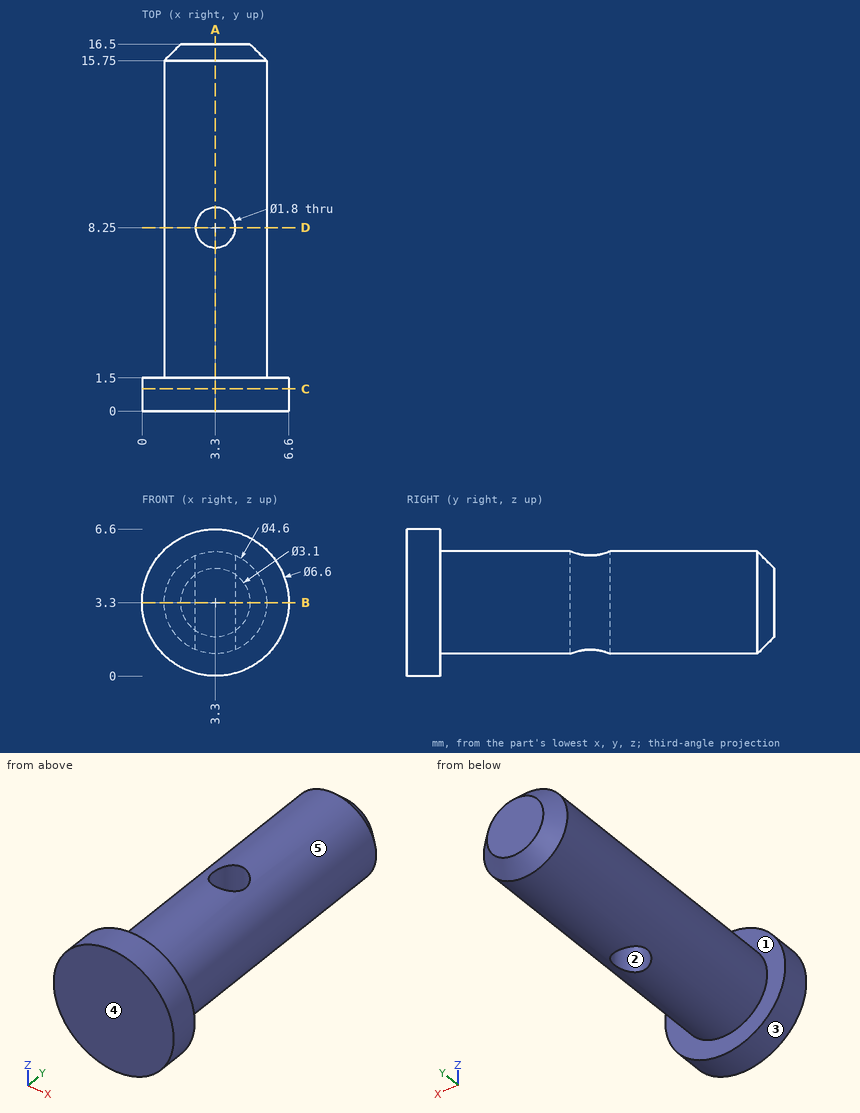
Study the drawing (mm; zero at the part's minimum x, y, z) and answer. A direction names the side the tool comes from. Coordinates: 2 decimals unless noted, no trailing zeros. Loops run counter-clockwise (first coordinate to the right, second up) from the corner with the lowest first, then second, coordinate; pieces in that order, holes last. Notation, with made-up numbers: M -11,-27 L 27,-27 A22 cw 27,-16 Z; hole C -15.5,12 d2. An arc over 180 degrees is marked long. Answer in a Markdown table with one row per item. Add a question column.
1. Find section B-B, the plane z = 3.3. Write down the section's boundary in (x, y).
2. Find section C-C, the plane y = 1. Write down the section's boundary in (x, z).
3. The mould has two halves that part along X. Classify the marked faces 1, 2 and 3: pulls with the +X half, pulls with the -X half, needs draft (parallel to the pull), parting line crosses it, or undercut.
4. Flat-ended cylindrical pins translate along their axes: P1, Ø1.5, axis at y = 14.5, z = 2.5, coming from the -X side; P2, Ø1.5, axis at x = 5, z = 3.5, coming from the +Y side; P3, Ø1.5, axis at y = 5.5, z = 0.5, coming from the -X side; P4, Ø2, axis at x = 4, y = 12, coming from the +Z side. Find the tip coordinate at first contact, or state that the pin passes through.
5. Find section A-A, the plane x = 3.3. Write down the section's boundary in (y, z).
6. Find section D-D, the plane y = 8.25. Write down the section's boundary in (x, z), then the cut area to 3 significant figures.
7. A tool of negligible diameter and unlimited length cuts with its end or side. For the marked faces 4 and 5, from which of +Z, -Z, +X, -X, +Y, -Y can it reach the whole face along a straight path? Write none if from no direction.
8. Consider L1, parallel to Y at x = 3.3, z = 4.3; L2, parallel to Y at x = 1, z = 2; L3, parallel to X at y = 7.75, z = 3. Determine where each line is inside the solid, lowest interval first.
Reported:
| question | item | result |
|---|---|---|
| 1 | outline | M 0,0 L 6.6,0 L 6.6,1.5 L 5.6,1.5 L 5.6,15.75 L 4.85,16.5 L 1.75,16.5 L 1,15.75 L 1,1.5 L 0,1.5 Z; hole C 3.3,8.25 d1.8 |
| 2 | outline | C 3.3,3.3 d6.6 |
| 3 | face 1 | needs draft |
| 3 | face 2 | undercut |
| 3 | face 3 | parting line crosses it |
| 4 | P1 | stops at x = 1 |
| 4 | P2 | stops at y = 16.5 |
| 4 | P3 | stops at x = 2.26 |
| 4 | P4 | stops at z = 5.6 |
| 5 | outline | M 0,0 L 1.5,0 L 1.5,1 L 7.35,1 L 7.35,5.6 L 1.5,5.6 L 1.5,6.6 L 0,6.6 Z; M 9.15,1 L 15.75,1 L 16.5,1.75 L 16.5,4.85 L 15.75,5.6 L 9.15,5.6 Z |
| 6 | outline | M 2.4,1.18 L 2.4,5.42 A2.3 ccw Z; M 4.2,1.18 A2.3 ccw 4.2,5.42 Z |
| 6 | area | 8.56 mm^2 |
| 7 | face 4 | +Z, -Z, +X, -X, -Y |
| 7 | face 5 | +Y |
| 8 | L1 | y = 0 to 7.35, 9.15 to 16.5 |
| 8 | L2 | y = 0 to 1.5 |
| 8 | L3 | x = 1.02 to 2.55, 4.05 to 5.58 |
